from build123d import *

# Parameters (mm, degrees)
F0_R     = 4
F1_DEPTH = 10
F3_DEPTH = 40
F4_R     = 3
F4_R_2   = 13.31729
F5_DEPTH = 25


with BuildPart() as f1:
    # F0 (on Front) → F1 (new body)
    with BuildSketch(Plane.XZ):
        Polygon((38.877375, 31.887809), (-31.122625, 31.887809), (-31.122625, 11.887809), (-16.122625, 11.887809), (23.877375, 11.887809), (38.877375, 11.887809), align=None)
        with Locations((-23.622625, 21.887809)):
            Circle(F0_R, mode=Mode.SUBTRACT)
        with Locations((31.377375, 21.887809)):
            Circle(F0_R, mode=Mode.SUBTRACT)
    extrude(amount=F1_DEPTH)

    # F2 (on face) → F3 (join)
    with BuildSketch(Plane.XZ.offset(10)):
        Polygon((-17.34383, 19.387809), (-16.122625, 19.387809), (23.877375, 19.387809), (24.928454, 19.387809), (24.928454, 24.387809), (23.877375, 24.387809), (-16.122625, 24.387809), (-17.34383, 24.387809), align=None)
    extrude(amount=F3_DEPTH)

    # F4 (on face) → F5 (cut)
    with BuildSketch(Plane(origin=(0, 0, 19.387809), x_dir=(1, 0, 0), z_dir=(0, 0, -1))):
        with Locations((20.653736, 14.044937)):
            Circle(F4_R)
        with Locations((-13.069112, 14.044937)):
            Circle(F4_R)
        with Locations((-13.069112, 45.955063)):
            Circle(F4_R)
        with Locations((20.653736, 45.955063)):
            Circle(F4_R)
        with Locations((3.792312, 30)):
            Circle(F4_R_2)
    extrude(amount=-F5_DEPTH, mode=Mode.SUBTRACT)


solid = f1.part
For this review, take the finished solid that the model builds, in its own axes (mm). A direction names the side the tool comes from. Coordinates: 2 decimals unless noted, no trailing zeros. Loops run counter-clockwise (first coordinate to the right, second up) from the corner with the lowest first, then second, coordinate; pieces in that order, holes last. Notation, with made-up numbers: (-3.5, -17.5) - (7.5, -17.5) arc R18 ccw to (7.5, 3.5) - close; hole circle Ø9 at (34, -4). An arc over 180 degrees is marked (long way). Use a Markdown table: item, result. Add a question column.
Item 1: We need section A-A (y = -30). Give the boundary of the cut face in (x, z), and give its area (3 significant figures).
Item 2: We need section B-B (x = 28.5). Give the boundary of the cut face in (y, z).
Item 3: Tool access review of faces 4 (the face through (-17.344, -30, 22)), 5 (the face through (4, -16, 24.388)), 6 (the face through (3, -16, 19.388)), 7 (the face through (24.928, -30, 22)): name each direction out of +Z, -Z, +X, -X, +Y, -Y from which nothing blocks a thin tool from reaching the whole face with its end or side.
Item 4: For line 1 (Y direction, x = -14.5, z = 21.75); line 2 (X direction, y = -9, z = 25.5); line 3 (X direction, y = -8.5, z = 23.25), list the stretches that pass through material, from the lowest coordinate up.
Item 5: Mouldability with a two-part tool opening along X and no side actions: class faces 1 (the face through (-31.123, -5, 22)), 2 (the face through (3, -50, 22)), 3 (the face through (20.003, -43.026, 21.853)) as pulls with the +X half, pulls with the -X half, needs draft (parallel to the pull), parting line crosses it, or undercut.
Item 6: Insertion check: pin 1 Ø5 at (x, y) = (-18, -28.5) entering from -Z; pin 2 Ø1.5 at (y, z) = (-31.5, 22.5) entering from +X; pin 3 Ø8 at (x, y) = (20.65, -14.04) entering from +Z; pin 4 Ø20 at (x, y) = (1.5, -30.5) entering from -Z. Each pin has a flat end and moves straight along its axis. Give the tip position at first contact, or say it passes through.
Item 7: We need section C-C (y = -12). Give the boundary of the cut face in (x, z).
Item 8: We need section D-D (x = -14.5). Give the boundary of the cut face in (y, z), and give its area (3 significant figures).
Results list:
| question | item | result |
|---|---|---|
| 1 | outline | (-17.34, 19.39) - (-9.52, 19.39) - (-9.52, 24.39) - (-17.34, 24.39) - close; (17.11, 19.39) - (24.93, 19.39) - (24.93, 24.39) - (17.11, 24.39) - close |
| 1 | area | 78.2 mm^2 |
| 2 | outline | (-10, 11.89) - (0, 11.89) - (0, 19.11) - (-10, 19.11) - close; (-10, 24.67) - (0, 24.67) - (0, 31.89) - (-10, 31.89) - close |
| 3 | face 4 | +Z, -Z, -X, -Y |
| 3 | face 5 | +Z, +X, -X, -Y |
| 3 | face 6 | -Z, +X, -X, -Y |
| 3 | face 7 | +Z, -Z, +X, -Y |
| 4 | line 1 | y = -50 to -48.59, -43.32 to -16.68, -11.41 to 0 |
| 4 | line 2 | x = -31.12 to -25.34, -21.9 to 29.66, 33.1 to 38.88 |
| 4 | line 3 | x = -31.12 to -27.38, -19.86 to 27.62, 35.14 to 38.88 |
| 5 | face 1 | pulls with the -X half |
| 5 | face 2 | needs draft |
| 5 | face 3 | undercut |
| 6 | pin 1 | stops at z = 19.39 |
| 6 | pin 2 | stops at x = 24.93 |
| 6 | pin 3 | stops at z = 24.39 |
| 6 | pin 4 | passes through |
| 7 | outline | (-17.34, 19.39) - (-15.26, 19.39) - (-15.26, 24.39) - (-17.34, 24.39) - close; (-10.87, 19.39) - (18.46, 19.39) - (18.46, 24.39) - (-10.87, 24.39) - close; (22.85, 19.39) - (24.93, 19.39) - (24.93, 24.39) - (22.85, 24.39) - close |
| 8 | outline | (-50, 19.39) - (-48.59, 19.39) - (-48.59, 24.39) - (-50, 24.39) - close; (-43.32, 19.39) - (-16.68, 19.39) - (-16.68, 24.39) - (-43.32, 24.39) - close; (-11.41, 19.39) - (-10, 19.39) - (-10, 11.89) - (0, 11.89) - (0, 31.89) - (-10, 31.89) - (-10, 24.39) - (-11.41, 24.39) - close |
| 8 | area | 347 mm^2 |
